Could you check a few things on this model? Use its own coordinates, in mm. A direction names the side the tool comes from. Round coordinates to 2 decimals unless told otherwise and drop trailing zeros. Write each loop counter-clockwise with the first axis right and the second up, starting at its lowest first coordinate (ties: lowest second). Pieces come first, ordered by that corner, then holes. Notation, with made-up numbers: (-29.75, 64) -> (-15.75, 64) arc R30 ccw to (-15.75, 95) -> close; hole circle Ø6 at (79.25, 9). An arc over 180 degrees is marked (long way). Answer as CSV lines item,"result". Start each with the question number.
Q1. Imagine slicing it at C-C on y = -24.5. Please give me the cut outline in (x, z).
Q2. Imagine slicing it at A-A on x = 11.5. Please give me the cut outline in (y, z).
Q3. Imagine slicing it at B-B on z = -105. Please give me the cut outline in (x, y), and give its area (4 significant figures).
Q4. Imagine slicing it at D-D on z = -29.5. Please give me the cut outline in (x, y).
Q5. If I drill on line 1 (Y direction, x = 0.9, z = 97.25); line 2 (Z direction, x = 14.75, y = -20); line 3 (Y direction, x = 6, z = 42.5), over which ranges is the centre line in solid material (lowest first)? Write a range as [from, to].
Q6. Will these pins go through, and if not, where does the flat tip stop? pin 1 Ø4 at (y, z) = (-4.08, -112.75) entering from +X; pin 2 Ø1.6 at (x, z) = (7, -134.5) entering from -Y; pin 3 Ø0.8 at (x, z) = (10, -134) entering from +Y.
Q7. If we mould it in two halves opening along Y, with no side actions, what happens to faces 4 (the flat face through (9, 36, 2)), 5 (the cylindrical face through (0.74, 34.49, 132.15)), 6 (the cylindrical face through (0.74, -34.49, -132.15)), 7 (the cylindrical face through (0.74, -24.236, 110.994))? For each: pulls with the +Y half, pulls with the -Y half, needs draft (parallel to the pull), parting line crosses it, or undercut.
Q8. For faces 1 (the flat face through (9, -36, -2)), 2 (the cylindrical face through (0.74, 34.65, -131.99)), 3 (the flat face through (11, 0, 133.5)), which set-ups out of +Z, -Z, +X, -X, +Y, -Y let a thin tool reach every point of the face, with its end or its side?
from build123d import *

# Parameters (mm, degrees)
SKETCH1_R           = 1.5
SKETCH1_R_2         = 6
BOSS_EXTRUDE1_DEPTH = 1.5
SKETCH2_W           = 1.5
SKETCH2_H           = 55
BOSS_EXTRUDE2_DEPTH = 15
SKETCH4_R           = 1.5
CUT_EXTRUDE1_DEPTH  = 10
SKETCH6_R           = 1.5
CUT_EXTRUDE2_DEPTH  = 76
SKETCH8_R           = 1.5
CUT_EXTRUDE3_DEPTH  = 271


with BuildPart() as part:
    # Sketch1 → Boss-Extrude1 (new body)
    with BuildSketch(Plane(origin=(0, 0, 0), x_dir=(0, 0, -1), z_dir=(1, 0, 0))):
        with BuildLine():
            Line((-125, 37.5), (125, 37.5))
            ThreePointArc((125, 37.5), (132.071067812, 34.571067812), (135, 27.5))
            Line((135, 27.5), (135, -27.5))
            ThreePointArc((135, -27.5), (132.071067812, -34.571067812), (125, -37.5))
            Line((125, -37.5), (-125, -37.5))
            ThreePointArc((-125, -37.5), (-132.071067812, -34.571067812), (-135, -27.5))
            Line((-135, -27.5), (-135, 27.5))
            ThreePointArc((-135, 27.5), (-132.071067812, 34.571067812), (-125, 37.5))
        make_face()
        with Locations((-112.75, -4.076606241)):
            Circle(SKETCH1_R, mode=Mode.SUBTRACT)
        with Locations((-120.5, -17.5)):
            Circle(SKETCH1_R, mode=Mode.SUBTRACT)
        with Locations((-97.25, -4.076606241)):
            Circle(SKETCH1_R, mode=Mode.SUBTRACT)
        with Locations((-105, -24.5)):
            Circle(SKETCH1_R_2, mode=Mode.SUBTRACT)
        with Locations((-89.5, -17.5)):
            Circle(SKETCH1_R, mode=Mode.SUBTRACT)
        with Locations((-97.25, -30.923393759)):
            Circle(SKETCH1_R, mode=Mode.SUBTRACT)
        with Locations((-112.75, -30.923393759)):
            Circle(SKETCH1_R, mode=Mode.SUBTRACT)
        with Locations((112.75, -30.923393759)):
            Circle(SKETCH1_R, mode=Mode.SUBTRACT)
        with Locations((120.5, -17.5)):
            Circle(SKETCH1_R, mode=Mode.SUBTRACT)
        with Locations((105, -24.5)):
            Circle(SKETCH1_R_2, mode=Mode.SUBTRACT)
        with Locations((97.25, -30.923393759)):
            Circle(SKETCH1_R, mode=Mode.SUBTRACT)
        with Locations((89.5, -17.5)):
            Circle(SKETCH1_R, mode=Mode.SUBTRACT)
        with Locations((97.25, -4.076606241)):
            Circle(SKETCH1_R, mode=Mode.SUBTRACT)
        with Locations((112.75, -4.076606241)):
            Circle(SKETCH1_R, mode=Mode.SUBTRACT)
    extrude(amount=BOSS_EXTRUDE1_DEPTH)

    # Sketch2 → Boss-Extrude2 (add)
    with BuildSketch(Plane(origin=(1.5, 0, 0), x_dir=(0, 0, -1), z_dir=(1, 0, 0))):
        Polygon((-90, 36), (-125, 36), (-125, 37.5), (-90, 37.5), (0, 37.5), (90, 37.5), (125, 37.5), (125, 36), (90, 36), align=None)
        Polygon((90, -37.5), (125, -37.5), (125, -36), (90, -36), (-90, -36), (-125, -36), (-125, -37.5), (-90, -37.5), align=None)
        with Locations((-134.25, 0)):
            Rectangle(SKETCH2_W, SKETCH2_H)
        with Locations((134.25, 0)):
            Rectangle(SKETCH2_W, SKETCH2_H)
    extrude(amount=BOSS_EXTRUDE2_DEPTH)

    # Sketch4 → Cut-Extrude1 (cut)
    with BuildSketch(Plane.ZY):
        with Locations((55, 20)):
            Circle(SKETCH4_R)
        with Locations((10, 20)):
            Circle(SKETCH4_R)
        with Locations((100, 20)):
            Circle(SKETCH4_R)
        with Locations((-10, 20)):
            Circle(SKETCH4_R)
        with Locations((-55, 20)):
            Circle(SKETCH4_R)
        with Locations((-100, 20)):
            Circle(SKETCH4_R)
    extrude(amount=-CUT_EXTRUDE1_DEPTH, mode=Mode.SUBTRACT)

    # Sketch6 → Cut-Extrude2 (cut, through all)
    with BuildSketch(Plane(origin=(0, 37.5, 0), x_dir=(1, 0, 0), z_dir=(0, 1, 0))):
        with Locations((7.5, 10)):
            Circle(SKETCH6_R)
        with Locations((7.5, -10)):
            Circle(SKETCH6_R)
        with Locations((7.5, 40)):
            Circle(SKETCH6_R)
        with Locations((7.5, 70)):
            Circle(SKETCH6_R)
        with Locations((7.5, 100)):
            Circle(SKETCH6_R)
        with Locations((7.5, -40)):
            Circle(SKETCH6_R)
        with Locations((7.5, -70)):
            Circle(SKETCH6_R)
        with Locations((7.5, -100)):
            Circle(SKETCH6_R)
    extrude(amount=-CUT_EXTRUDE2_DEPTH, mode=Mode.SUBTRACT)

    # Sketch8 → Cut-Extrude3 (cut, through all)
    with BuildSketch(Plane.XY.offset(135)):
        with Locations((7.5, 15)):
            Circle(SKETCH8_R)
        with Locations((7.5, 0)):
            Circle(SKETCH8_R)
        with Locations((7.5, -15)):
            Circle(SKETCH8_R)
    extrude(amount=-CUT_EXTRUDE3_DEPTH, mode=Mode.SUBTRACT)


solid = part.part
Checks:
1,outline,"(0, -135) -> (16.5, -135) -> (16.5, -133.5) -> (1.5, -133.5) -> (1.5, -111) -> (0, -111) -> close; (0, -99) -> (1.5, -99) -> (1.5, 99) -> (0, 99) -> close; (0, 111) -> (1.5, 111) -> (1.5, 133.5) -> (16.5, 133.5) -> (16.5, 135) -> (0, 135) -> close"
2,outline,"(-37.5, -125) -> (-36, -125) -> (-36, 125) -> (-37.5, 125) -> close; (-27.5, -135) -> (27.5, -135) -> (27.5, -133.5) -> (-27.5, -133.5) -> close; (-27.5, 133.5) -> (27.5, 133.5) -> (27.5, 135) -> (-27.5, 135) -> close; (36, -125) -> (37.5, -125) -> (37.5, 125) -> (36, 125) -> close"
3,outline,"(0, -37.5) -> (16.5, -37.5) -> (16.5, -36) -> (1.5, -36) -> (1.5, -30.5) -> (0, -30.5) -> close; (0, -18.5) -> (1.5, -18.5) -> (1.5, 36) -> (16.5, 36) -> (16.5, 37.5) -> (0, 37.5) -> close"
3,area,"139.5 mm^2"
4,outline,"(0, -37.5) -> (16.5, -37.5) -> (16.5, -36) -> (1.5, -36) -> (1.5, 36) -> (16.5, 36) -> (16.5, 37.5) -> (0, 37.5) -> close"
5,line 1,"[-37.5, -32.42], [-29.42, -5.58], [-2.58, 37.5]"
5,line 2,"[-135, -133.5], [133.5, 135]"
5,line 3,"[-37.5, -36], [36, 37.5]"
6,pin 1,"x = 1.5"
6,pin 2,"y = -27.5"
6,pin 3,"y = 27.5"
7,face 4,"undercut"
7,face 5,"pulls with the +Y half"
7,face 6,"pulls with the -Y half"
7,face 7,"undercut"
8,face 1,"+Z, -Z, +X"
8,face 2,"-Z, +X, -X, +Y"
8,face 3,"+X, +Y, -Y"
